Geometry check sheet. Reference: the model listing, model coordinates, mm. Face numbers are marked on the shaded views. A direction names the side the tool comes from. Coordinates: 2 decimals unless noted, no trailing zeros. Write each loop counter-clockwise with the first axis right and the second up, starting at its lowest first coordinate (ties: lowest second). Pieces come first, ordered by that corner, then holes. Notation, with made-up numbers: (86.25, 36.25) - (139.25, 36.25) arc R14 cw to (139.25, 59.25) - close; hole circle Ø11 at (-5, 87). An arc over 180 degrees is marked (long way). Answer as a JSON object with one key per item and string values. Group by question number.
from build123d import *

# Parameters (mm, degrees)
SKETCH1_W           = 55
SKETCH1_H           = 55
BOSS_EXTRUDE1_DEPTH = 30
SKETCH2_R           = 21.25
CUT_EXTRUDE1_DEPTH  = 30
SKETCH3_W           = 41
SKETCH3_H           = 16
CUT_EXTRUDE2_DEPTH  = 60
SKETCH4_W           = 16
SKETCH4_H           = 41
CUT_EXTRUDE3_DEPTH  = 60
SKETCH5_R           = 2.125
CUT_EXTRUDE4_DEPTH  = 10


with BuildPart() as part:
    # Sketch1 → Boss-Extrude1 (new body)
    with BuildSketch(Plane.XY):
        Rectangle(SKETCH1_W, SKETCH1_H)
    extrude(amount=BOSS_EXTRUDE1_DEPTH)

    # Sketch2 → Cut-Extrude1 (cut)
    with BuildSketch(Plane.XY.offset(30)):
        Circle(SKETCH2_R)
    extrude(amount=-CUT_EXTRUDE1_DEPTH, mode=Mode.SUBTRACT)

    # Sketch3 → Cut-Extrude2 (cut)
    with BuildSketch(Plane(origin=(0, 27.5, 0), x_dir=(1, 0, 0), z_dir=(0, 1, 0))):
        with Locations((0, -15)):
            Rectangle(SKETCH3_W, SKETCH3_H)
    extrude(amount=-CUT_EXTRUDE2_DEPTH, mode=Mode.SUBTRACT)

    # Sketch4 → Cut-Extrude3 (cut)
    with BuildSketch(Plane(origin=(27.5, 0, 0), x_dir=(0, 0, -1), z_dir=(1, 0, 0))):
        with Locations((-15, 0)):
            Rectangle(SKETCH4_W, SKETCH4_H)
    extrude(amount=-CUT_EXTRUDE3_DEPTH, mode=Mode.SUBTRACT)

    # Sketch5 → Cut-Extrude4 (cut)
    with BuildSketch(Plane(origin=(0, 27.5, 0), x_dir=(1, 0, 0), z_dir=(0, 1, 0))):
        with Locations(Location((-24, -14, 0), (0, 0, 270))):
            Circle(SKETCH5_R)
        with Locations(Location((24, -14, 0), (0, 0, 270))):
            Circle(SKETCH5_R)
    extrude(amount=-CUT_EXTRUDE4_DEPTH, mode=Mode.SUBTRACT)


solid = part.part
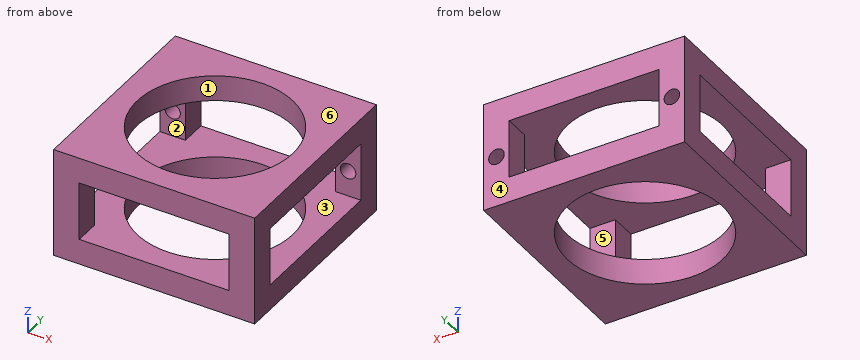
(1) Set-up check for the marked faces 1, 2 and 3: record each of +Z, -Z, +X, -X, +Y, -Y from which the full face is reachable in a straight line by a thin tool's end or side.
(2) Gauge pin test, flat end, axial feed: pin 1 (7 mm diameter, centred on x = 24, z = 14, fed in from +Y). Record the tip position at first contact, or that the pin passes through.
(3) Section check C-C (z = 14). Record the cut outline in (x, y) (3 decimals).
(4) Section check D-D (x = -24). Record the cut outline in (y, z) (3 decimals).
(5) Section check B-B (y = 0). Record the cut outline in (x, z).
(6) Draft check along Y on the marked faces 4, 5 and 6. Enter one of: +Y half, -Y half, draft (parallel to the pull), parting line (faces both ways), or undercut.
(7) Material ranges on L1, parallel to X at y = 26.25, z = 14 (3 decimals); L2, parallel to Z at x = -19, y = -10.5; L3, parallel to Y at x = 0, z = 27.75, recorded low to high. Write a range as [from, to].
(8) Section check A-A (x = 17). Record the cut outline in (y, z).
Conclusion:
{
 "1": {"face 1": "+Z, -Z", "face 2": "+X, -X", "face 3": "none"},
 "2": {"pin 1": "stops at y = 27.5"},
 "3": {"outline": "(-27.5, -27.5) - (-20.5, -27.5) - (-20.5, -20.5) - (-27.5, -20.5) - close; (-27.5, 20.5) - (-26.125, 20.5) - (-26.125, 27.5) - (-27.5, 27.5) - close; (-21.875, 20.5) - (-20.5, 20.5) - (-20.5, 27.5) - (-21.875, 27.5) - close; (20.5, -27.5) - (27.5, -27.5) - (27.5, -20.5) - (20.5, -20.5) - close; (20.5, 20.5) - (21.875, 20.5) - (21.875, 27.5) - (20.5, 27.5) - close; (26.125, 20.5) - (27.5, 20.5) - (27.5, 27.5) - (26.125, 27.5) - close"},
 "4": {"outline": "(-27.5, 0) - (27.5, 0) - (27.5, 11.875) - (20.5, 11.875) - (20.5, 7) - (-20.5, 7) - (-20.5, 23) - (20.5, 23) - (20.5, 16.125) - (27.5, 16.125) - (27.5, 30) - (-27.5, 30) - close"},
 "5": {"outline": "(-27.5, 0) - (-21.25, 0) - (-21.25, 7) - (-27.5, 7) - close; (-27.5, 23) - (-21.25, 23) - (-21.25, 30) - (-27.5, 30) - close; (21.25, 0) - (27.5, 0) - (27.5, 7) - (21.25, 7) - close; (21.25, 23) - (27.5, 23) - (27.5, 30) - (21.25, 30) - close"},
 "6": {"face 4": "+Y half", "face 5": "undercut", "face 6": "draft"},
 "7": {"L1": "x = [-27.5, -26.125], [-21.875, -20.5], [20.5, 21.875], [26.125, 27.5]", "L2": "z = [0, 7], [23, 30]", "L3": "y = [-27.5, -21.25], [21.25, 27.5]"},
 "8": {"outline": "(-27.5, 0) - (-12.75, 0) - (-12.75, 7) - (-27.5, 7) - close; (-27.5, 23) - (-12.75, 23) - (-12.75, 30) - (-27.5, 30) - close; (12.75, 0) - (27.5, 0) - (27.5, 7) - (12.75, 7) - close; (12.75, 23) - (27.5, 23) - (27.5, 30) - (12.75, 30) - close"}
}
